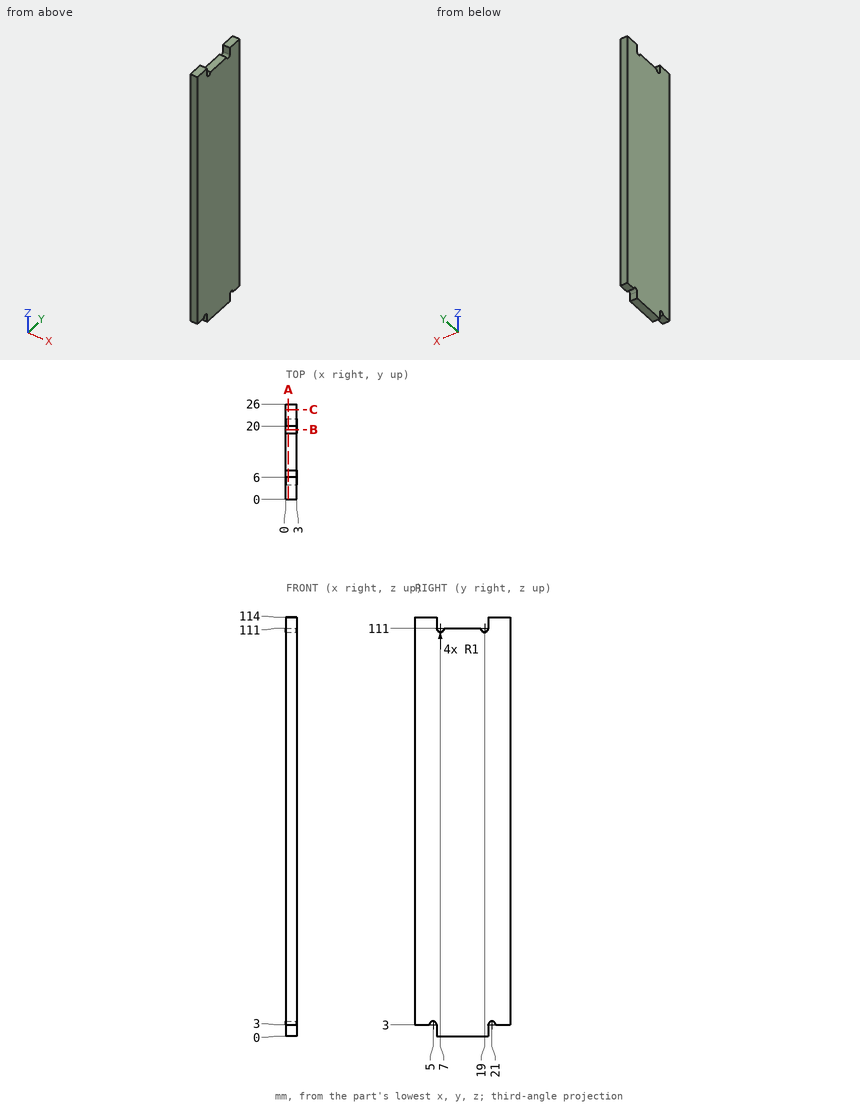
The figure shows three views and two pictorial views of one solid part (mm, origin at its lowest corner). Answer the questions. Round coordinates to 2 decimals unless told otherwise and drop trailing zeros. Loops run counter-clockwise (first coordinate to the right, second up) from the corner with the lowest first, then second, coordinate; pieces in that order, holes last. Notation, with made-up numbers: (42, 34) - (88, 34) arc R25 ccw to (88, 65) - close; hole circle Ø8 at (9.25, 43.25). An arc over 180 degrees is marked (long way). One line per question, with ' | ' between items. Start each with the question number.
Q1. Section A-A on x = 0.7 is taken. Give the vertices of the cut face in (y, z), plus the area to 3 significant figures.
Q2. Flat-ended cylindrical pins translate along their axes: pin 1 (0.9 mm diameter, centred on x = 1.5, y = 13, fed in from +Z); pin 2 (1.5 mm diameter, centred on x = 2, z = 2, fed in from +Y); pin 3 (1.5 mm diameter, centred on x = 1.5, y = 2.5, fed in from -Z). Find the tip coordinate at first contact, or state that the pin passes through.
Q3. Section B-B on y = 19 is taken. Give the vertices of the cut face in (x, z).
Q4. Section C-C on y = 24.5 is taken. Give the vertices of the cut face in (x, z).
Q5. Find the intervals of material crossed by L1, parallel to Z at x = 1.35, y = 24.5; L2, parallel to Z at x = 1.8, y = 12.25, in increasing order.
Established:
1) outline: (0, 3) - (4, 3) arc R1 cw to (6, 3) - (6, 0) - (20, 0) - (20, 3) arc R1 cw to (22, 3) - (26, 3) - (26, 114) - (20, 114) - (20, 111) arc R1 cw to (18, 111) - (8, 111) arc R1 cw to (6, 111) - (6, 114) - (0, 114) - close | area: 2,880 mm²
2) pin 1: z = 111 | pin 2: y = 20 | pin 3: z = 3
3) outline: (0, 0) - (3, 0) - (3, 110) - (0, 110) - close
4) outline: (0, 3) - (3, 3) - (3, 114) - (0, 114) - close
5) L1: 3 to 114 | L2: 0 to 111
